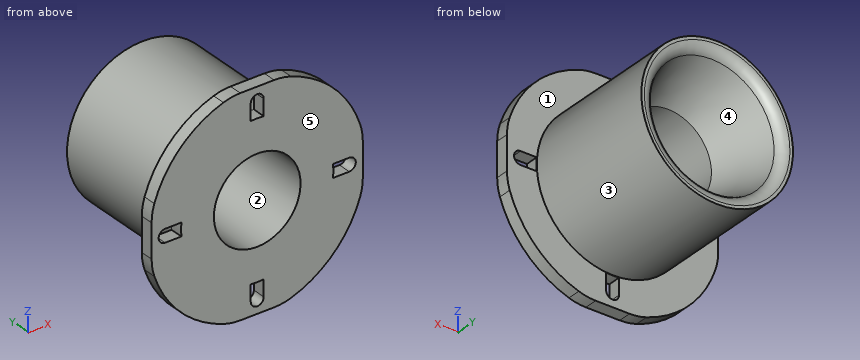
```python
from build123d import *

# Parameters (mm, degrees)
FILLET1_R           = 2.54
BOSS_EXTRUDE1_START = -3.048
SKETCH2_R           = 25.4
SKETCH2_R_2         = 17.78
BOSS_EXTRUDE1_DEPTH = 3.048
CUT_EXTRUDE1_START  = -3.048
CUT_EXTRUDE1_DEPTH  = 3.048
SKETCH5_OUTSIDE_W   = 68.832
SKETCH5_OUTSIDE_H   = 68.832
SKETCH5_OUTSIDE_W_2 = 49.53
SKETCH5_OUTSIDE_H_2 = 49.53
CUT_EXTRUDE2_DEPTH  = 49.449459687
FILLET2_R           = 12.7


# Read off the part's stored shape, not the designer's step: Cut-Extrude1
with BuildPart() as part:
    # Sketch1 → Revolve1 (revolve)
    with BuildSketch(Plane(origin=(0, 0, 0), x_dir=(0, 0, -1), z_dir=(1, 0, 0)), mode=Mode.PRIVATE) as revolve1_sk:
        Polygon((-15.24, 0), (-10.16, -15.24), (-10.16, -35.56), (-17.78, -35.56), (-17.78, 0), align=None)
    revolve(revolve1_sk.sketch.rotate(Axis((0, -35.56, 0), (0, 1, 0)), 180), axis=Axis((0, -35.56, 0), (0, 1, 0)))

    # Fillet1
    fillet1_edges = [part.edges().sort_by_distance(p)[0] for p in [
        (0, 0, 15.24),
    ]]
    fillet(fillet1_edges, radius=FILLET1_R)

    # Sketch2 → Boss-Extrude1 (add)
    with BuildSketch(Plane.XZ.offset(35.56).offset(BOSS_EXTRUDE1_START)):
        with Locations(Location((0, 0, 0), (0, 0, 270))):
            Circle(SKETCH2_R)
        with Locations(Location((0, 0, 0), (0, 0, 270))):
            Circle(SKETCH2_R_2, mode=Mode.SUBTRACT)
    extrude(amount=BOSS_EXTRUDE1_DEPTH)

    # Cut-Extrude1 outline → Cut-Extrude1 (cut)
    with BuildSketch(Plane(origin=(0, -32.512, 0), x_dir=(1, 0, 0), z_dir=(0, 1, 0)).offset(CUT_EXTRUDE1_START)):
        with BuildLine():
            ThreePointArc((-1.524, 17.78), (0, 17.845194759), (1.524, 17.78))
            Line((1.524, 17.78), (1.524, 21.59))
            ThreePointArc((1.524, 21.59), (0, 23.114), (-1.524, 21.59))
            Line((-1.524, 21.59), (-1.524, 17.78))
        make_face()
        with BuildLine():
            ThreePointArc((-17.78, -1.524), (-17.845194759, 0), (-17.78, 1.524))
            Line((-17.78, 1.524), (-21.59, 1.524))
            ThreePointArc((-21.59, 1.524), (-23.114, 0), (-21.59, -1.524))
            Line((-21.59, -1.524), (-17.78, -1.524))
        make_face()
        with BuildLine():
            ThreePointArc((1.524, -17.78), (0, -17.845194759), (-1.524, -17.78))
            Line((-1.524, -17.78), (-1.524, -21.59))
            ThreePointArc((-1.524, -21.59), (0, -23.114), (1.524, -21.59))
            Line((1.524, -21.59), (1.524, -17.78))
        make_face()
        with BuildLine():
            ThreePointArc((17.78, 1.524), (17.845194759, 0), (17.78, -1.524))
            Line((17.78, -1.524), (21.59, -1.524))
            ThreePointArc((21.59, -1.524), (23.114, 0), (21.59, 1.524))
            Line((21.59, 1.524), (17.78, 1.524))
        make_face()
    extrude(amount=CUT_EXTRUDE1_DEPTH, mode=Mode.SUBTRACT)

    # Sketch5 outside → Cut-Extrude2 (cut, through all)
    with BuildSketch(Plane(origin=(0, -32.512, 0), x_dir=(1, 0, 0), z_dir=(0, 1, 0))):
        Rectangle(SKETCH5_OUTSIDE_W, SKETCH5_OUTSIDE_H)
        Rectangle(SKETCH5_OUTSIDE_W_2, SKETCH5_OUTSIDE_H_2, mode=Mode.SUBTRACT)
    extrude(amount=-CUT_EXTRUDE2_DEPTH, mode=Mode.SUBTRACT)

    # Fillet2
    fillet2_edges = [part.edges().sort_by_distance(p)[0] for p in [
        (24.765, -34.036, 5.644003455),
        (24.765, -34.036, -5.644003455),
        (-5.644003455, -34.036, 24.765),
        (5.644003455, -34.036, 24.765),
        (-24.765, -34.036, -5.644003455),
        (-24.765, -34.036, 5.644003455),
        (5.644003455, -34.036, -24.765),
        (-5.644003455, -34.036, -24.765),
    ]]
    fillet(fillet2_edges, radius=FILLET2_R)


solid = part.part
```
Model file for the job. Use its own axes, mm. Face numbers are marked on the shaded views. A direction names the side the tool comes from. Round coordinates to 2 decimals unless told otherwise and drop trailing zeros. Loops run counter-clockwise (first coordinate to the right, second up) from the corner with the lowest first, then second, coordinate; pieces in that order, holes last. Notation, with made-up numbers: M 24,-3 L 30,-3 A20 ccw 30,34 Z; hole C -7.5,15 d7. An arc over 180 degrees is marked long. Put each result on its own line as item: value. Start each with the question number.
Item 1: Cut at C-C (y = -29.5). List the corners of the cut face in (x, z), then the cut area to 3 significant figures.
Item 2: Drop flat-ended pins along their axis: P1, Ø12, axis at y = -31, z = 15.5, coming from the +X side; P2, Ø3.5, axis at y = -34.5, z = 19.5, coming from the -X side; P3, Ø3.5, axis at x = -20, y = -33.5, coming from the +Z side; P4, Ø10, axis at x = -1.5, z = -1.5, coming from the -Y side. Give the stop position or say it passes through.
Item 3: Cut at D-D (y = -3). List the corners of the cut face in (x, z).
Item 4: Drill centre lines: line 1 along X through (y, z) = (-23.25, 0); line 2 along Y through (x, z) = (21.5, -2.5); line 3 along Z through (x, y) = (-5, -15). Where is each one in solid material? Low to high.
Item 5: Cut at A-A (x = 0). List the corners of the cut face in (y, z) (3 decimals), then the cut area to 3 significant figures.
Item 6: Cut at B-B (z = 0). List the corners of the cut face in (x, y) (3 decimals), then the cut area to 3 significant figures.
Item 7: 3-axis set-ups, long thin cutter, end or side, ignore diameter. For the marked faces 1 and 2: which of +Z, -Z, +X, -X, +Y, -Y reach the whole face in a straight line?
Item 8: Mould opens along Z. For the marked faces 3, 4 and 5 say: released by +Z, released by -Z, zero draft, split by the parting line, or undercut.
Answer block:
1. outline: C 0,0 d35.56; hole C 0,0 d20.32
1. area: 669 mm2
2. P1: x = 23.48
2. P2: x = -18.17
2. P3: z = 17.67
2. P4: through
3. outline: C 0,0 d35.56; hole C 0,0 d28.48
4. line 1: -17.78 to -10.16, 10.16 to 17.78
4. line 2: -35.56 to -32.51
4. line 3: -17.06 to -8.94, 8.94 to 17.06
5. outline: M -35.56,-24.765 L -32.512,-24.765 L -32.512,-23.114 L -35.56,-23.114 Z; M -35.56,-17.845 L -32.512,-17.845 L -32.512,-17.78 L 0,-17.78 L 0,-17.071 A2.54 ccw -1.737,-14.661 L -15.24,-10.16 L -35.56,-10.16 Z; M -35.56,10.16 L -15.24,10.16 L -1.737,14.661 A2.54 ccw 0,17.071 L 0,17.78 L -32.512,17.78 L -32.512,17.845 L -35.56,17.845 Z; M -35.56,23.114 L -32.512,23.114 L -32.512,24.765 L -35.56,24.765 Z
5. area: 474 mm2
6. outline: M -24.765,-35.56 L -23.114,-35.56 L -23.114,-32.512 L -24.765,-32.512 Z; M -17.845,-35.56 L -10.16,-35.56 L -10.16,-15.24 L -14.661,-1.737 A2.54 ccw -17.071,0 L -17.78,0 L -17.78,-32.512 L -17.845,-32.512 Z; M 10.16,-35.56 L 17.845,-35.56 L 17.845,-32.512 L 17.78,-32.512 L 17.78,0 L 17.071,0 A2.54 ccw 14.661,-1.737 L 10.16,-15.24 Z; M 23.114,-35.56 L 24.765,-35.56 L 24.765,-32.512 L 23.114,-32.512 Z
6. area: 474 mm2
7. face 1: +Y
7. face 2: +Y, -Y
8. face 3: split by the parting line
8. face 4: undercut
8. face 5: zero draft
